Model file for the job. Use its own axes, mm. Round coordinates to 2 decimals unless told otherwise and drop trailing zeros. Write each loop counter-clockwise with the first axis right and the second up, starting at its lowest first coordinate (ties: lowest second). Pieces come first, ordered by that corner, then holes. Notation, with made-up numbers: (-25.75, 59) - (1.25, 59) arc R24 ccw to (1.25, 85) - close; hole circle Ø3 at (29, -8). An arc over 180 degrees is marked (long way). Answer as a JSON object with one key per item and string values. Group by question number.
from build123d import *

# Parameters (mm, degrees)
BOSS_EXTRUDE1_DEPTH               = 3.175
SKETCH2_W                         = 2.75
SKETCH2_H                         = 2.5
SKETCH2_H_2                       = 4
SKETCH2_W_2                       = 1.125
SKETCH2_H_3                       = 7.5
CUT_EXTRUDE1_DEPTH                = 204.460831631
CIRPATTERN1_COUNT                 = 2
CIRPATTERN1_ANGLE                 = 65
CIRPATTERN1_THE_OTHER_WAY_COUNT   = 2
CIRPATTERN1_THE_OTHER_WAY_ANGLE   = 65
F_3_0_3_DIAMETER_HOLE1_D          = 3
SKETCH13_W                        = 6.35
SKETCH13_H                        = 33.16
CUT_EXTRUDE2_DEPTH                = 204.530492207
M2_5X0_45_TAPPED_HOLE1_AT_2_COUNT = 2
M2_5X0_45_TAPPED_HOLE1_AT_2_PITCH = 16.83
M6_CLEARANCE_HOLE1_D              = 7


with BuildPart() as part:
    # Sketch1 → Boss-Extrude1 (new, symmetric)
    with BuildSketch(Plane(origin=(0, 0, 0), x_dir=(1, 0, 0), z_dir=(0, 1, 0))):
        with BuildLine():
            Line((88.95, 33.202731801), (138.254290129, 56.193699868))
            ThreePointArc((138.254290129, 56.193699868), (0, 149.238), (-138.254290129, 56.193699868))
            Line((-138.254290129, 56.193699868), (-58.85, 19.16687129))
            Line((-58.85, 19.16687129), (-58.85, -38.1))
            Line((-58.85, -38.1), (88.95, -38.1))
            Line((88.95, -38.1), (88.95, 33.202731801))
        make_face()
        with BuildLine():
            Line((-7.5, 11.821590418), (-7.5, 11.772641828))
            Line((-7.5, 11.772641828), (-7.544362488, 11.793328396))
            ThreePointArc((-7.544362488, 11.793328396), (-7.522194517, 11.807480241), (-7.5, 11.821590418))
        make_face(mode=Mode.SUBTRACT)
        with BuildLine():
            ThreePointArc((7.5, 11.821590418), (7.522194517, 11.807480241), (7.544362488, 11.793328396))
            Line((7.544362488, 11.793328396), (7.5, 11.772641828))
            Line((7.5, 11.772641828), (7.5, 11.821590418))
        make_face(mode=Mode.SUBTRACT)
        with BuildLine():
            Line((-7.5, 134.028320306), (-7.5, 38.1))
            Line((-7.5, 38.1), (-58.85, 38.1))
            Line((-58.85, 38.1), (-58.85, 35.717540075))
            Line((-58.85, 35.717540075), (-118.301273414, 63.440124154))
            ThreePointArc((-118.301273414, 63.440124154), (-72.126024825, 113.215180903), (-7.5, 134.028320306))
        make_face(mode=Mode.SUBTRACT)
        with BuildLine():
            ThreePointArc((7.5, 134.028320306), (72.126024825, 113.215180903), (118.301273414, 63.440124154))
            Line((118.301273414, 63.440124154), (63.959201798, 38.1))
            Line((63.959201798, 38.1), (7.5, 38.1))
            Line((7.5, 38.1), (7.5, 134.028320306))
        make_face(mode=Mode.SUBTRACT)
    extrude(amount=BOSS_EXTRUDE1_DEPTH, both=True)

    # Sketch2 → Cut-Extrude1 (cut, symmetric)
    with BuildSketch(Plane(origin=(0, 0, 0), x_dir=(1, 0, 0), z_dir=(0, 1, 0))):
        with Locations((0, 136.488)):
            Rectangle(SKETCH2_W, SKETCH2_H)
        with Locations((0, 139.738)):
            Rectangle(SKETCH2_W, SKETCH2_H_2)
        with Locations((1.9375, 139.738)):
            Rectangle(SKETCH2_W_2, SKETCH2_H_2)
        with Locations((0, 145.488)):
            Rectangle(SKETCH2_W, SKETCH2_H_3)
        with Locations((-1.9375, 139.738)):
            Rectangle(SKETCH2_W_2, SKETCH2_H_2)
    cut_extrude1 = extrude(amount=CUT_EXTRUDE1_DEPTH, both=True, mode=Mode.SUBTRACT)

    # CirPattern1: Cut-Extrude1 ×2 about axis
    cirpattern1_axis = Axis((0, 0, 0), (0, 1, 0))
    for i in range(1, CIRPATTERN1_COUNT):
        add(cut_extrude1.rotate(cirpattern1_axis, i * CIRPATTERN1_ANGLE / (CIRPATTERN1_COUNT - 1)), mode=Mode.SUBTRACT)

    # CirPattern1 the other way: Cut-Extrude1 ×2 about axis
    cirpattern1_the_other_way_axis = Axis((0, 0, 0), (0, -1, 0))
    for i in range(1, CIRPATTERN1_THE_OTHER_WAY_COUNT):
        add(cut_extrude1.rotate(cirpattern1_the_other_way_axis, i * CIRPATTERN1_THE_OTHER_WAY_ANGLE / (CIRPATTERN1_THE_OTHER_WAY_COUNT - 1)), mode=Mode.SUBTRACT)

    # Ø3.0 (3) Diameter Hole1 (through all)
    with Locations(Plane(origin=(0, 3.175, 0), x_dir=(1, 0, 0), z_dir=(0, 1, 0))):
        with Locations((76.155771888, 119.540616747), (-76.155771888, 119.540616747)):
            Hole(F_3_0_3_DIAMETER_HOLE1_D / 2)

    # Sketch13 → Cut-Extrude2 (cut, through all)
    with BuildSketch(Plane(origin=(0, 3.175, 0), x_dir=(1, 0, 0), z_dir=(0, 1, 0))):
        with Locations((-55.675, 0)):
            Rectangle(SKETCH13_W, SKETCH13_H)
        with Locations((85.775, 0)):
            Rectangle(SKETCH13_W, SKETCH13_H)
    extrude(amount=-CUT_EXTRUDE2_DEPTH, mode=Mode.SUBTRACT)

    # Sketch15 → M2.5x0.45 Tapped Hole1 (revolve, cut)
    with BuildSketch(Plane(origin=(-52.5, 0, -8.415), x_dir=(0, 0, 1), z_dir=(0, 1, 0))):
        Polygon((0, 0), (0, 6.965882135), (1.025, 6.35), (1.025, 0), align=None)
    m2_5x0_45_tapped_hole1 = revolve(axis=Axis((-58.85, 0, -8.415), (1, 0, 0)), mode=Mode.SUBTRACT)

    # M2.5x0.45 Tapped Hole1 at 2: M2.5x0.45 Tapped Hole1 ×2
    with Locations(*[(0, 0, i * M2_5X0_45_TAPPED_HOLE1_AT_2_PITCH) for i in range(1, M2_5X0_45_TAPPED_HOLE1_AT_2_COUNT)]):
        add(m2_5x0_45_tapped_hole1, mode=Mode.SUBTRACT)

    # Mirror1: M2.5x0.45 Tapped Hole1 across plane
    add(m2_5x0_45_tapped_hole1.mirror(Plane.ZY.offset(-15.05)), mode=Mode.SUBTRACT)

    # Mirror1 copy 1 sketch → Mirror1 copy 1 (revolve, cut)
    with BuildSketch(Plane(origin=(82.6, 0, 8.415), x_dir=(0, 0, 1), z_dir=(0, 1, 0))):
        Polygon((0, 0), (0, -6.965882135), (1.025, -6.35), (1.025, 0), align=None)
    revolve(axis=Axis((88.95, 0, 8.415), (1, 0, 0)), mode=Mode.SUBTRACT)

    # M6 Clearance Hole1 (through all)
    with Locations(Plane(origin=(0, 3.175, 0), x_dir=(1, 0, 0), z_dir=(0, 1, 0))):
        with Locations((99.909557827, 46.588591938), (-95.378018892, 44.475500629)):
            Hole(M6_CLEARANCE_HOLE1_D / 2)


solid = part.part
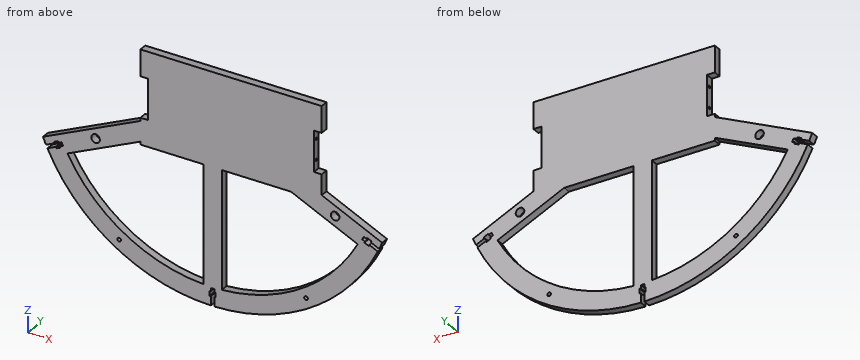
(1) Slice it at B-B (z = -71.5). Write the cut outline in (x, y) (3 decimals), then the cut area to 3 significant figures.
(2) Slice it at A-A (x = -86). Write the cut outline in (y, z) (3 decimals), then the cut area to 3 significant figures.
(3) Flat gauge pins, fed straight in: pin 1 (3 mm diameter, centred on x = 90.5, y = 1.5, fed in from -Z); pin 2 (1.9 mm diameter, centred on y = 1.5, z = 23, fed in from +X); pin 3 (2 mm diameter, centred on x = 105, y = 0, fed in from +Z). Where does each tip first touch, or does it go through?
(4) Slice it at C-C (z = -2.5). Write the cut outline in (x, y) (3 decimals), then the cut area to 3 significant figures.
(5) Drill centre lines: line 1 (X direction, y = 2.75, z = -109.5); line 2 (X direction, y = -1.5, z = -53.5); line 3 (X direction, y = 2.25, z = -59.5). Where is each one in solid material? Low to high. Write a range as from..to.
(6) Slice it at D-D (x = 25). Write the cut outline in (y, z) (1 decimal).
Answer:
{
 "1": {"outline": "(-130.995, -3.175) - (-113.612, -3.175) - (-113.612, 3.175) - (-130.995, 3.175) - close; (-7.5, -3.175) - (7.5, -3.175) - (7.5, 3.175) - (-7.5, 3.175) - close; (113.612, -3.175) - (130.995, -3.175) - (130.995, 3.175) - (113.612, 3.175) - close", "area": "316 mm²"},
 "2": {"outline": "(-3.175, -121.967) - (3.175, -121.967) - (3.175, -103.072) - (-3.175, -103.072) - close; (-3.175, -48.378) - (3.175, -48.378) - (3.175, -31.827) - (-3.175, -31.827) - close", "area": "225 mm²"},
 "3": {"pin 1": "z = -119.8", "pin 2": "x = 88.95", "pin 3": "z = -40.22"},
 "4": {"outline": "(-52.5, -3.175) - (82.6, -3.175) - (82.6, 3.175) - (-52.5, 3.175) - close", "area": "858 mm²"},
 "5": {"line 1": "-101.4..-77.65, -7.5..7.5, 77.65..101.4", "line 2": "-132.48..-96.98, -7.5..7.5, 96.98..132.48", "line 3": "-136.86..-130.85, -124.23..-109.85, -7.5..7.5, 109.85..124.23, 130.85..136.86"},
 "6": {"outline": "(-3.2, -147.1) - (3.2, -147.1) - (3.2, -131.9) - (-3.2, -131.9) - close; (-3.2, -38.1) - (3.2, -38.1) - (3.2, 38.1) - (-3.2, 38.1) - close"}
}
